Can you work these out from the model? Positions are in its coordinate system, mm. Face numbers are marked on the shaded views. A direction names the side the tool comes from. Coordinates: 2 decimals unless noted, no trailing zeros. Order: outer loops, then holes, each group sorted by start corner. A loop starts at its lowest first (then second) coordinate and runs counter-clockwise, first axis right, second up. Notation, with made-up numbers: M 72.25,-32.75 L 104.25,-32.75 A18 ccw 104.25,-5.75 Z; hole C 11,86.25 d9. An arc over 180 degrees is marked long. Answer as a JSON object with one key per item and string values.
from build123d import *

# Parameters (mm, degrees)
SKETCH1_R           = 12
BOSS_EXTRUDE1_DEPTH = 8
FILLET2_R           = 6
SKETCH2_R           = 2.1
CUT_EXTRUDE1_DEPTH  = 34.763886032
FILLET3_DEPTH       = 8
FILLET4_R           = 3


with BuildPart() as part:
    # Sketch1 → Boss-Extrude1 (new body)
    with BuildSketch(Plane(origin=(0, 0, 0), x_dir=(1, 0, 0), z_dir=(0, 1, 0))):
        with BuildLine():
            Line((0, -15), (6, -15))
            Line((6, -15), (11, -13))
            Line((11, -13), (26, -13))
            Line((26, -13), (26, -5))
            Line((26, -5), (15, -5))
            Line((15, -5), (15, 0))
            ThreePointArc((15, 0), (-10.606601718, 10.606601718), (0, -15))
        make_face()
        with Locations(Location((0, 0, 0), (0, 0, 270))):
            Circle(SKETCH1_R, mode=Mode.SUBTRACT)
    extrude(amount=BOSS_EXTRUDE1_DEPTH)

    # Fillet2
    fillet2_edges = [part.edges().sort_by_distance(p)[0] for p in [
        (11, 4, 13),
        (6, 4, 15),
    ]]
    fillet(fillet2_edges, radius=FILLET2_R)

    # Sketch2 → Cut-Extrude1 (cut, through all)
    with BuildSketch(Plane(origin=(0, 0, 5), x_dir=(-1, 0, 0), z_dir=(0, 0, -1))):
        with Locations((-22, 4)):
            Circle(SKETCH2_R)
    extrude(amount=-CUT_EXTRUDE1_DEPTH, mode=Mode.SUBTRACT)

    # Fillet3: read off the stored shape, not the designer's step
    # Fillet3 outline → Fillet3 (add)
    with BuildSketch(Plane(origin=(0, 0, 0), x_dir=(1, 0, 0), z_dir=(0, 1, 0))):
        with BuildLine():
            Line((15, -5), (18.973665961, -5))
            add(Edge.make_bspline(
                [(18.973665961, -5), (15.284342024, -5), (14.979209969, 0.789473684)],
                knots=[0, 0, 0, 1, 1, 1], degree=2, weights=[1, 0.72547625, 1]))
            ThreePointArc((14.979209969, 0.789473684), (14.994801592, 0.39487369), (15, 0))
            Line((15, 0), (15, -5))
        make_face()
    extrude(amount=FILLET3_DEPTH)

    # Fillet4
    fillet4_edges = [part.edges().sort_by_distance(p)[0] for p in [
        (26, 0, 9),
        (26, 8, 9),
    ]]
    fillet(fillet4_edges, radius=FILLET4_R)


solid = part.part
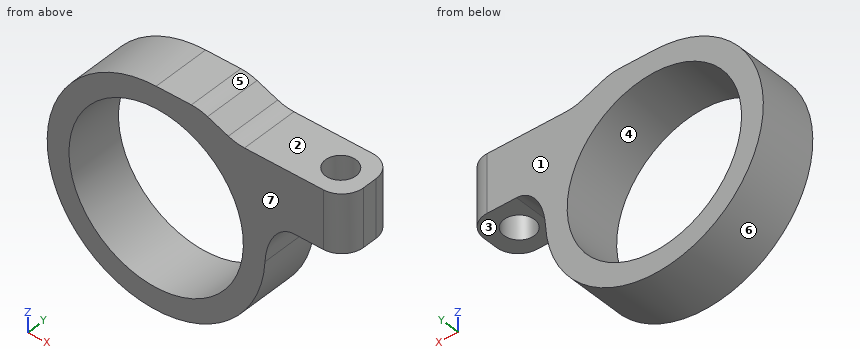
Item 1: I want a section at B-B, the plane y = 4. Give the number of separate pieces and of enclosed holes in the cut face, plus the area to 3 significant figures.
Answers follow:
{"separate pieces": "2", "enclosed holes": "1", "area": "349 mm^2"}
Item 2: I want a section at A-A, the plane x = -6.5. Write out the boundary of the cut face in (y, z), plus the area to 3 significant figures.
Answers follow:
{"outline": "M 0,-13.52 L 8,-13.52 L 8,-10.09 L 0,-10.09 Z; M 0,10.09 L 8,10.09 L 8,13.52 L 0,13.52 Z", "area": "54.9 mm^2"}
Item 3: Which directions (+Z, -Z, +X, -X, +Y, -Y) give clear straight access to the entire face, cutting with the end or side of a thin tool? Please do the marked faces 1, 2 and 3.
Answers follow:
{"face 1": "+Z, -Z, +X, -X, +Y", "face 2": "+Z, +X, +Y, -Y", "face 3": "-Z, +X, +Y, -Y"}
Item 4: I'm going to push flat-ended pins straight in: pin 1 (4 mm diameter, centred on y = 1.5, z = 11, fed in from -X); pin 2 (4 mm diameter, centred on x = 19, y = 4, fed in from +Z); pin 3 (4 mm diameter, centred on x = 22, y = 4, fed in from +Z); pin 4 (1 mm diameter, centred on x = -4.5, y = 3, fed in from -Z). Where does each tip first touch, or does it pass through?
Answers follow:
{"pin 1": "stops at x = -12", "pin 2": "stops at z = 13", "pin 3": "passes through", "pin 4": "stops at z = -14.46"}
Item 5: I want a section at C-C, the plane x = -1.5. Write out the boundary of the cut face in (y, z).
Answers follow:
{"outline": "M 0,-14.92 L 8,-14.92 L 8,-11.91 L 0,-11.91 Z; M 0,11.91 L 8,11.91 L 8,14.92 L 0,14.92 Z"}
Item 6: I want a section at D-D, the plane z = -13. Write out the boundary of the cut face in (x, y).
Answers follow:
{"outline": "M -7.48,0 L 7.48,0 L 7.48,8 L -7.48,8 Z"}
Item 7: Please list where these lines run through material, in increasing order: line 1 (Y direction, x = 22, z = 11.5); line 2 (X direction, y = 3, z = 5.5); line 3 (X direction, y = 5, z = -10).
Answers follow:
{"line 1": "y = 0 to 1.9, 6.1 to 8", "line 2": "x = -13.96 to -10.67, 10.67 to 20.15, 23.85 to 26", "line 3": "x = -11.18 to -6.63, 6.63 to 11.18"}
Item 8: If we mould it in two halves opening along X, with no side actions, what happens to the marked faces 4, 5, 6 and 7? For each: pulls with the +X half, pulls with the -X half, needs draft (parallel to the pull), parting line crosses it, or undercut.
Answers follow:
{"face 4": "undercut", "face 5": "pulls with the +X half", "face 6": "parting line crosses it", "face 7": "needs draft"}
